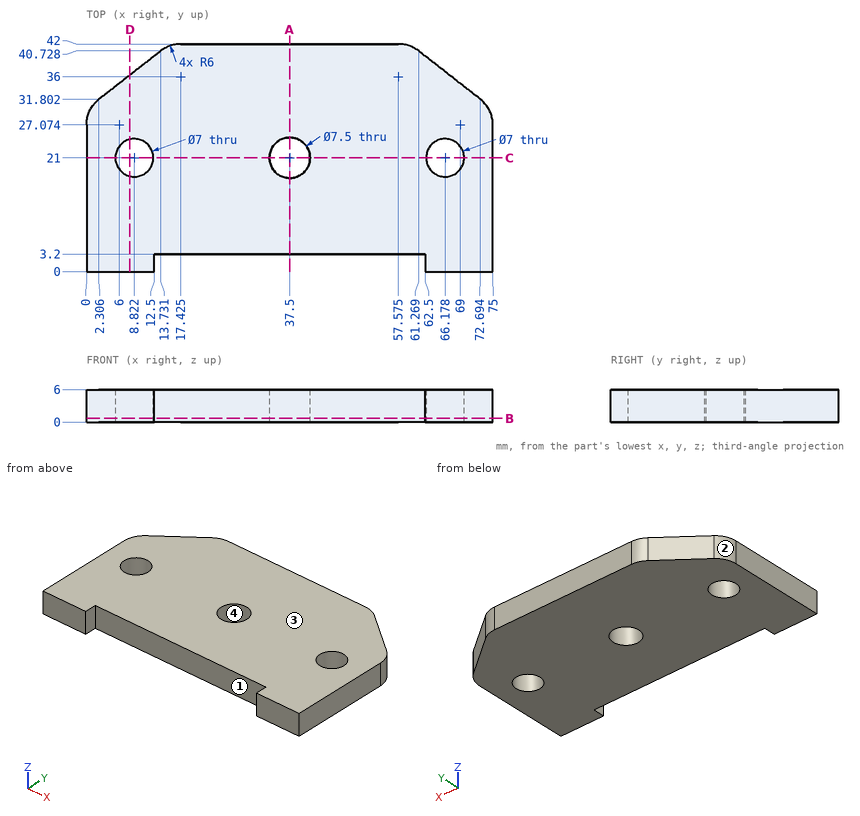
Can you work these out from the drawing? Everything is in mm from the part's minimum corner. Give positions to 0.01 mm unless a question says otherwise; leave off trailing zeros. Write each loop counter-clockwise with the first axis right and the second up, starting at its lowest first coordinate (ties: lowest second). Pieces come first, ordered by that corner, then holes. Notation, with made-up numbers: M 66.25,13 L 76.25,13 A26 ccw 76.25,30 Z; hole C 23.25,13 d5. An arc over 180 degrees is marked long. Answer in a Markdown table with one row per item. Add a question column.
Item 1: Imagine slicing it at A-A, the plane x = 37.5. Write out the boundary of the cut face in (y, z).
Item 2: Imagine slicing it at B-B, the plane z = 0.7. State how many separate pieces and enclosed holes the cut face has, plus the area to 3 significant figures.
Item 3: Imagine slicing it at D-D, the plane x = 8. Write out the boundary of the cut face in (y, z), plus the area to 3 significant figures.
Item 4: Imagine slicing it at C-C, the plane y = 21. Write out the boundary of the cut face in (x, z), plus the area to 3 significant figures.
Item 5: For pin 1 Ø11 at (x, y) = (66.178, 21) entering from -Z; pin 2 Ø3 at (x, z) = (49.5, 4) entering from -Y, each with a flat end and sliding along its axis, tell me the tip position at first contact or that it passes through.
Item 6: We'd pull the mould along X, two halves only. Please class the marked faces 1, 2, 3 and 4: released by +X, released by -X, zero draft, split by the parting line, or undercut.
Item 7: Please list where these lines run through material, in increasing order: L1, parallel to Y at x = 37.5, z = 1.75; L2, parallel to Y at x = 52.5, z = 2.5; L3, parallel to Y at x = 34.5, z = 2.95.
Evaluation:
| question | item | result |
|---|---|---|
| 1 | outline | M 3.2,0 L 17.25,0 L 17.25,6 L 3.2,6 Z; M 24.75,0 L 42,0 L 42,6 L 24.75,6 Z |
| 2 | separate pieces | 1 |
| 2 | enclosed holes | 3 |
| 2 | area | 2,680 mm² |
| 3 | outline | M 0,0 L 17.6,0 L 17.6,6 L 0,6 Z; M 24.4,0 L 36.25,0 L 36.25,6 L 24.4,6 Z |
| 3 | area | 177 mm² |
| 4 | outline | M 0,0 L 5.32,0 L 5.32,6 L 0,6 Z; M 12.32,0 L 33.75,0 L 33.75,6 L 12.32,6 Z; M 41.25,0 L 62.68,0 L 62.68,6 L 41.25,6 Z; M 69.68,0 L 75,0 L 75,6 L 69.68,6 Z |
| 4 | area | 321 mm² |
| 5 | pin 1 | stops at z = 0 |
| 5 | pin 2 | stops at y = 3.2 |
| 6 | face 1 | undercut |
| 6 | face 2 | released by -X |
| 6 | face 3 | zero draft |
| 6 | face 4 | undercut |
| 7 | L1 | y = 3.2 to 17.25, 24.75 to 42 |
| 7 | L2 | y = 3.2 to 42 |
| 7 | L3 | y = 3.2 to 18.75, 23.25 to 42 |
